```python
from build123d import *

# Parameters (mm, degrees)
REVOLUTION001_ANGLE = 55
REVOLUTION_ANGLE    = -190


with BuildPart() as right_pillar_round_down:
    # Sketch093 → Revolution001 (revolve)
    with BuildSketch(Plane(origin=(17.15, 72.5, 3), x_dir=(1, 0, 0), z_dir=(0, -1, 0))):
        with BuildLine():
            ThreePointArc((-3.895747, 0), (-3.191385, 0.294392), (-2.899991, 1))
            Line((-2.899991, 1), (-2.5, 1))
            Line((-2.5, 1), (-2.5, 0))
            Line((-3.895747, 0), (-2.5, 0))
        make_face()
    revolve(axis=Axis((17.15, 72.5, 3), (0, 0, 1)), revolution_arc=REVOLUTION001_ANGLE)


with BuildPart() as pillar_right_custom_round_base:
    # Sketch092 → Revolution (revolve)
    with BuildSketch(Plane(origin=(17.15, 72.5, 3), x_dir=(1, 0, 0), z_dir=(0, -1, 0))):
        with BuildLine():
            ThreePointArc((-3.895747, 0), (-3.191385, 0.294392), (-2.899991, 1))
            Line((-2.899991, 1), (-2.5, 1))
            Line((-2.5, 1), (-2.5, 0))
            Line((-3.895747, 0), (-2.5, 0))
        make_face()
    revolve(axis=Axis((17.15, 72.5, 3), (0, 0, 1)), revolution_arc=REVOLUTION_ANGLE)

    # Fusion007039: union right_pillar_round_down
    add(right_pillar_round_down.part)


solid = pillar_right_custom_round_base.part
```
Can you work these out from the model? Positions are in its coordinate system, mm. Coordinates: 2 decimals unless noted, no trailing zeros. Loops run counter-clockwise (first coordinate to the right, second up) from the corner with the lowest first, then second, coordinate; pieces in that order, holes last.
1) Thinking about a two-plate mould opening in Y: for faces 1 (the flat face through (16, 75, 3)), 2 (the cylindrical face through (16.263, 74.837, 3.493)), 3 (the flat face through (19.98, 72, 3.4)), which applies, pulls with the +Y half, pulls with the -Y half, needs draft (parallel to the pull), parting line crosses it, or undercut?
2) Imagine slicing it at C-C on z = 3.2. List the corners of the cut face in (x, y) for me, plus the area to 3 significant figures.
3) Imagine slicing it at B-B on x = 17.15. List the corners of the cut face in (y, z) for me, plus the area to 3 significant figures.
4) Imagine slicing it at A-A on y = 72.5. List the corners of the cut face in (x, z) for me.
5) I need wall thicknesses on probe 1 along Y at (x, z) = (16, 3.55); probe 2 along X at (y, z) = (72.5, 3.35); probe 3 along X at (y, z) = (71.5, 3.45). Which ranges of each line are inside material? Lowest first, please.
Completed:
1. face 1: needs draft
1. face 2: undercut
1. face 3: pulls with the -Y half
2. outline: (15.26, 69.8) - (15.72, 70.45) arc R2.5 cw (long way) to (19.61, 72.07) - (20.4, 71.93) arc R3.3 ccw (long way) to start
2. area: 9.92 mm2
3. outline: (75, 3) - (76.4, 3) arc R1 cw to (75.4, 4) - (75, 4) - close
3. area: 0.615 mm2
4. outline: (13.25, 3) - (14.65, 3) - (14.65, 4) - (14.25, 4) arc R1 cw to start; (19.65, 3) - (21.05, 3) arc R1 cw to (20.05, 4) - (19.65, 4) - close
5. probe 1: y = 74.72 to 75.28
5. probe 2: x = 14.01 to 14.65, 19.65 to 20.29
5. probe 3: x = 14.25 to 14.86
